Read the model definition and answer for the solid it produces. Units are mm, in the model's axes. Face numbers are marked on the shaded views. Coordinates: 2 decimals unless noted, no trailing zeros. Loops run counter-clockwise (first coordinate to the right, second up) from the corner with the lowest first, then second, coordinate; pieces in that order, holes last. Notation, with made-up numbers: (-25.5, 29.25) -> (-18.5, 29.25) arc R28 ccw to (-18.5, 58.25) -> close; hole circle Ø11 at (11.5, 77.5). An arc over 180 degrees is marked (long way). Answer as CSV lines item,"result".
```python
from build123d import *

# Parameters (mm, degrees)
SKETCH_1_R      = 2
EXTRUDE_1_DEPTH = 1
FILLET_1_R      = 2
FILLET_2_R      = 0.5
EXTRUDE_START   = -5.75
SKETCH_2_R      = 2.5
SKETCH_2_R_2    = 1.5
EXTRUDE_2_DEPTH = 6.75
EXTRUDE_START_2 = 12.5
SKETCH_2_3_R    = 2.5
SKETCH_2_3_R_2  = 1.5
EXTRUDE_3_DEPTH = 6.75


with BuildPart() as part:
    # 草图1 → 凸台-拉伸1 (new body)
    with BuildSketch(Plane(origin=(0, 0, 0), x_dir=(1, 0, 0), z_dir=(0, 1, 0))):
        Polygon((-5.75, 0), (-5.75, 1), (5.75, 1), (5.75, 0), (12.5, 0), (12.5, 1), (12.5, 12), (-12.5, 12), (-12.5, 1), (-12.5, 0), align=None)
        with Locations(Location((-7.5, 7.5, 0), (0, 0, 270))):
            Circle(SKETCH_1_R, mode=Mode.SUBTRACT)
        with Locations(Location((7.5, 7.5, 0), (0, 0, 270))):
            Circle(SKETCH_1_R, mode=Mode.SUBTRACT)
    extrude(amount=EXTRUDE_1_DEPTH)

    # 圆角1
    fillet_1_edges = [part.edges().sort_by_distance(p)[0] for p in [
        (-12.5, 0.5, -12),
        (12.5, 0.5, -12),
    ]]
    fillet(fillet_1_edges, radius=FILLET_1_R)

    # 圆角2
    fillet_2_edges = [part.edges().sort_by_distance(p)[0] for p in [
        (5.75, 0.5, -1),
        (-5.75, 0.5, -1),
    ]]
    fillet(fillet_2_edges, radius=FILLET_2_R)

    # 草图2 → 凸台-拉伸2 (add)
    with BuildSketch(Plane(origin=(0, 0, 0), x_dir=(0, 0, -1), z_dir=(1, 0, 0)).offset(EXTRUDE_START)):
        with Locations((-1.5, 2)):
            Circle(SKETCH_2_R)
        with Locations((-1.5, 2)):
            Circle(SKETCH_2_R_2, mode=Mode.SUBTRACT)
    extrude(amount=-EXTRUDE_2_DEPTH)

    # 草图2<3> → 凸台-拉伸3 (add)
    with BuildSketch(Plane(origin=(0, 0, 0), x_dir=(0, 0, -1), z_dir=(1, 0, 0)).offset(EXTRUDE_START_2)):
        with Locations((-1.5, 2)):
            Circle(SKETCH_2_3_R)
        with Locations((-1.5, 2)):
            Circle(SKETCH_2_3_R_2, mode=Mode.SUBTRACT)
    extrude(amount=-EXTRUDE_3_DEPTH)


solid = part.part
```
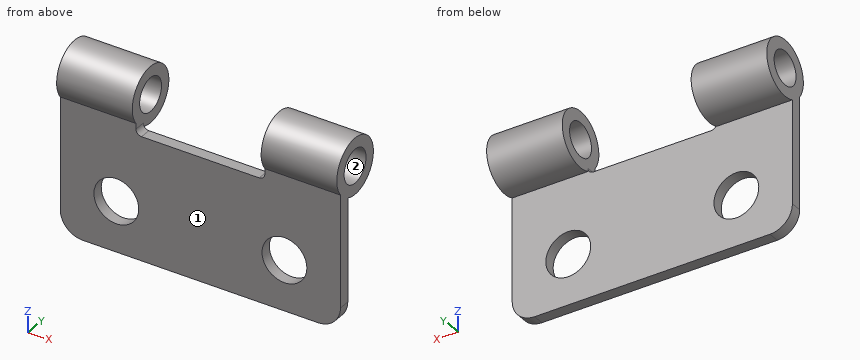
Q1. Given pin 1 Ø0.8 at (x, y) = (-0.5, 0.5) entering from +Z; pin 2 Ø1 at (x, z) = (-5, -2.5) entering from -Y; pin 3 Ø5 at (x, z) = (-7.5, -7.5) entering from +Y, each flat-ended and moving along its own axis, determine where each tip first touches the part or whether it passes through.
Results:
pin 1,"stops at z = -1"
pin 2,"stops at y = 0"
pin 3,"stops at y = 1"
Q2. For a pull along Y with two mould halves and no side action, classify the marked faces 1 and 2 as pulls with the +Y half, pulls with the -Y half, needs draft (parallel to the pull), parting line crosses it, or undercut.
Results:
face 1,"pulls with the -Y half"
face 2,"undercut"
Q3. A cutting plane is placed at B-B, the plane z = 1.5. Write down the section's boundary in (x, y), and give its area (3 significant figures).
Results:
outline,"(-12.5, -0.5) -> (-5.75, -0.5) -> (-5.75, 0.5) -> (-12.5, 0.5) -> close; (-12.5, 3.5) -> (-5.75, 3.5) -> (-5.75, 4.5) -> (-12.5, 4.5) -> close; (5.75, -0.5) -> (12.5, -0.5) -> (12.5, 0.5) -> (5.75, 0.5) -> close; (5.75, 3.5) -> (12.5, 3.5) -> (12.5, 4.5) -> (5.75, 4.5) -> close"
area,"27.0 mm²"
Q4. A cutting plane is placed at A-A, the plane y = 2. Write down the section's boundary in (x, z).
Results:
outline,"(-12.5, -1) -> (-5.75, -1) -> (-5.75, 0) -> (-12.5, 0) -> close; (-12.5, 3) -> (-5.75, 3) -> (-5.75, 4) -> (-12.5, 4) -> close; (5.75, -1) -> (12.5, -1) -> (12.5, 0) -> (5.75, 0) -> close; (5.75, 3) -> (12.5, 3) -> (12.5, 4) -> (5.75, 4) -> close"
Q5. Find the intervals of material crossed by probe 1 along X at (y, z) = (0.3, -7.5); probe 2 along Y at (x, z) = (10, 1.5); probe 3 along X at (y, z) = (1, 3.5), in increasing order. Write a range as [from, to].
Results:
probe 1,"x = [-12.5, -9.5], [-5.5, 5.5], [9.5, 12.5]"
probe 2,"y = [-0.5, 0.5], [3.5, 4.5]"
probe 3,"x = [-12.5, -5.75], [5.75, 12.5]"
Q6. A cutting plane is placed at D-D, the plane z = -8.5. Write down the section's boundary in (x, y), and give its area (3 significant figures).
Results:
outline,"(-12.5, 0) -> (-9.23, 0) -> (-9.23, 1) -> (-12.5, 1) -> close; (-5.77, 0) -> (5.77, 0) -> (5.77, 1) -> (-5.77, 1) -> close; (9.23, 0) -> (12.5, 0) -> (12.5, 1) -> (9.23, 1) -> close"
area,"18.1 mm²"
Q7. A cutting plane is placed at C-C, the plane x = -7.75. Write down the section's boundary in (y, z), and give its area (3 significant figures).
Results:
outline,"(0, -12) -> (1, -12) -> (1, -9.48) -> (0, -9.48) -> close; (0, -5.52) -> (1, -5.52) -> (1, -0.79) arc R2.5 ccw (long way) to (0, 0) -> close; hole circle Ø3 at (2, 1.5)"
area,"20.1 mm²"
